Model file for the job. Use its own axes, mm. Face numbers are marked on the shaded views. Round coordinates to 2 decimals unless told otherwise and drop trailing zeros. Loops run counter-clockwise (first coordinate to the right, second up) from the corner with the lowest first, then second, coordinate; pieces in that order, holes last. Notation, with made-up numbers: (-24, -13) -> (22, -13) arc R10 cw to (22, -2) -> close; hole circle Ø7 at (-2, -28). An arc over 180 degrees is marked (long way). Use a Markdown table: item, result. Add a question column.
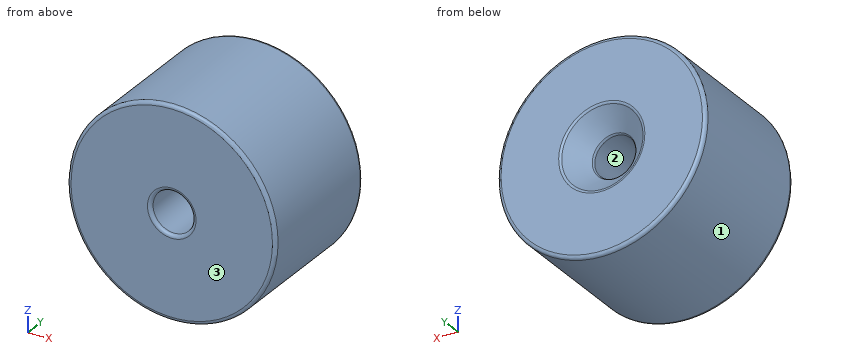
```python
from build123d import *

# Parameters (mm, degrees)
SKETCH1_R           = 15
SKETCH1_R_2         = 3
BOSS_EXTRUDE1_DEPTH = 20
CHAMFER1_SIZE       = 3
FILLET1_R           = 0.5


with BuildPart() as part:
    # Sketch1 → Boss-Extrude1 (new body)
    with BuildSketch(Plane(origin=(0, 0, 0), x_dir=(1, 0, 0), z_dir=(0, 1, 0))):
        with Locations(Location((0, 0, 0), (0, 0, 270))):
            Circle(SKETCH1_R)
        with Locations(Location((0, 0, 0), (0, 0, 270))):
            Circle(SKETCH1_R_2, mode=Mode.SUBTRACT)
    extrude(amount=BOSS_EXTRUDE1_DEPTH)

    # Chamfer1
    chamfer1_edges = [part.edges().sort_by_distance(p)[0] for p in [
        (0, 20, -3),
    ]]
    chamfer(chamfer1_edges, length=CHAMFER1_SIZE)

    # Fillet1
    fillet1_edges = [part.edges().sort_by_distance(p)[0] for p in [
        (0, 0, -15),
        (0, 20, -15),
        (0, 0, -3),
        (0, 17, -3),
        (0, 20, -6),
    ]]
    fillet(fillet1_edges, radius=FILLET1_R)


solid = part.part
```
1) Wall check: probe 1 along X at (y, z) = (11.25, 0); probe 2 along X at (y, z) = (17.5, -2); probe 3 along Z at (x, y) = (-2.5, 4.25). Give the ranges that are in metal, low to high. Write a range as from..to.
2) Cut at A-A on y = 2.75. Write the cut outline in (x, z).
3) Pin check, flat tips, straight feed: pin 1 Ø2 at (x, y) = (10.5, 2) entering from -Z; pin 2 Ø12 at (y, z) = (15, 10.5) entering from +X; pin 3 Ø1.5 at (y, z) = (10.5, 10.5) entering from +X. Stop position of each tip, or through.
4) Pull direction X, two halves, no side cores. Call the marked faces 1, 2 and 3: +X half, -X half, draft (parallel to the pull), parting line (faces both ways), or undercut.
Established:
| question | item | result |
|---|---|---|
| 1 | probe 1 | x = -15..-3, 3..15 |
| 1 | probe 2 | x = -14.87..-2.87, 2.87..14.87 |
| 1 | probe 3 | z = -14.79..-1.66, 1.66..14.79 |
| 2 | outline | circle Ø30 at (0, 0); hole circle Ø6 at (0, 0) |
| 3 | pin 1 | stops at z = -11.61 |
| 3 | pin 2 | stops at x = 14.31 |
| 3 | pin 3 | stops at x = 11.4 |
| 4 | face 1 | parting line |
| 4 | face 2 | undercut |
| 4 | face 3 | draft |
